```python
from build123d import *

# Parameters (mm, degrees)
F0_R     = 4.045
F0_R_2   = 1.575
F1_DEPTH = 5.44
F2_R     = 2.735
F3_DEPTH = 1.45
F4_R     = 2.375
F5_DEPTH = 2.5
F7_DEPTH = 2.4


with BuildPart() as f1:
    # F0 (on Front) → F1 (new body)
    with BuildSketch(Plane.XZ):
        Circle(F0_R)
        Circle(F0_R_2, mode=Mode.SUBTRACT)
    extrude(amount=F1_DEPTH)

    # F2 (on face) → F3 (cut)
    with BuildSketch(Plane.XZ.offset(5.44)):
        Circle(F2_R)
    extrude(amount=-F3_DEPTH, mode=Mode.SUBTRACT)

    # F4 (on face) → F5 (cut)
    with BuildSketch(Plane(origin=(0, 0, 0), x_dir=(-1, 0, 0), z_dir=(0, 1, 0))):
        Circle(F4_R)
    extrude(amount=-F5_DEPTH, mode=Mode.SUBTRACT)

    # F6 (on face) → F7 (join)
    with BuildSketch(Plane(origin=(0, 0, 0), x_dir=(-1, 0, 0), z_dir=(0, 1, 0))):
        with BuildLine():
            Line((1.4963533031, -0.268314818), (2.2665058776, -0.7096309653))
            ThreePointArc((2.2665058776, -0.7096309653), (2.3477197937, -0.3589383936), (2.375, 0))
            ThreePointArc((2.375, 0), (2.342926602, 0.3889986346), (2.247572684, 0.7674907361))
            Line((2.247572684, 0.7674907361), (1.4963533031, 0.266433459))
            ThreePointArc((1.4963533031, 0.266433459), (1.520064106, -0.0009406795), (1.4963533031, -0.268314818))
        make_face()
        with BuildLine():
            ThreePointArc((-0.7096309653, -2.2665058776), (0.0304393614, -2.3748049278), (0.7674907361, -2.247572684))
            Line((0.7674907361, -2.247572684), (0.266433459, -1.4963533031))
            ThreePointArc((0.266433459, -1.4963533031), (-0.0009406795, -1.520064106), (-0.268314818, -1.4963533031))
            Line((-0.268314818, -1.4963533031), (-0.7096309653, -2.2665058776))
        make_face()
        with BuildLine():
            ThreePointArc((-2.2665058776, 0.7096309653), (-2.3748049278, -0.0304393614), (-2.247572684, -0.7674907361))
            Line((-2.247572684, -0.7674907361), (-1.4963533031, -0.266433459))
            ThreePointArc((-1.4963533031, -0.266433459), (-1.520064106, 0.0009406795), (-1.4963533031, 0.268314818))
            Line((-1.4963533031, 0.268314818), (-2.2665058776, 0.7096309653))
        make_face()
        with BuildLine():
            ThreePointArc((0.7096309653, 2.2665058776), (-0.0304393614, 2.3748049278), (-0.7674907361, 2.247572684))
            Line((-0.7674907361, 2.247572684), (-0.266433459, 1.4963533031))
            ThreePointArc((-0.266433459, 1.4963533031), (0.0009406795, 1.520064106), (0.268314818, 1.4963533031))
            Line((0.268314818, 1.4963533031), (0.7096309653, 2.2665058776))
        make_face()
    extrude(amount=-F7_DEPTH)


solid = f1.part
```
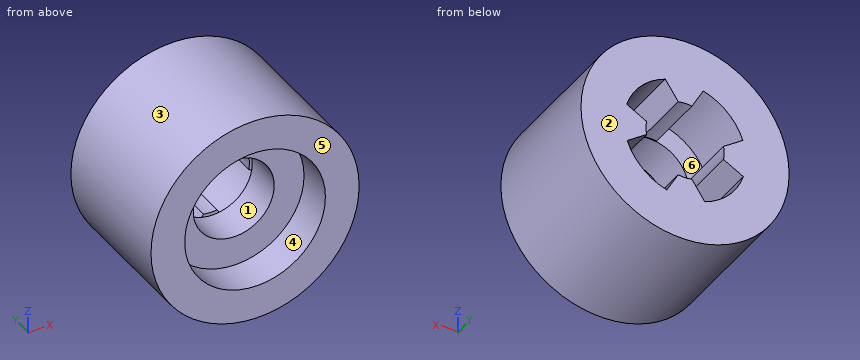
The listing builds one solid part. Answer for the finished solid, in the listing's coordinates (mm). Face numbers are marked on the shaded views. A direction names the side the tool comes from. Give positions to 0.01 mm unless a question says otherwise; leave off trailing zeros. Loops run counter-clockwise (first coordinate to the right, second up) from the corner with the lowest first, then second, coordinate; pieces in that order, holes last. Notation, with made-up numbers: M -2.5,82.5 L 15.5,82.5 A17 ccw 15.5,102.5 Z; hole C 28.5,-18 d8. An arc over 180 degrees is marked long. One line per item, written item: value.
Q1. Flat-ended cylindrical pins translate along their axes: P1, Ø3, axis at x = -2.5, y = -2.5, coming from the +Z side; P2, Ø1, axis at y = -4.5, z = -2, coming from the +X side; P3, Ø4.5, axis at x = 0, z = 0, coming from the -Y side. Find the tip coordinate at first contact, or state that the pin passes through.
Working result:
P1: stops at z = 3.92
P2: stops at x = 3.76
P3: stops at y = -3.99
Q2. A cutting plane is placed at B-B on x = 0. Determine the outline of the cut face in (y, z) (3 decimals).
Working result:
outline: M -5.44,-4.045 L 0,-4.045 L 0,-1.52 L -2.4,-1.52 L -2.4,-2.375 L -2.5,-2.375 L -2.5,-1.575 L -3.99,-1.575 L -3.99,-2.735 L -5.44,-2.735 Z; M -5.44,2.735 L -3.99,2.735 L -3.99,1.575 L -2.5,1.575 L -2.5,2.375 L -2.4,2.375 L -2.4,1.52 L 0,1.52 L 0,4.045 L -5.44,4.045 Z
Q3. For the marked faces 4, 5 and 6, determine the directions among +Z, -Z, +X, -X, +Y, -Y from which every point of the face is accessible in a straight line to the end or side of a thin tool.
Working result:
face 4: -Y
face 5: +Z, -Z, +X, -X, -Y
face 6: none
Q4. A cutting plane is placed at D-D on z = 2. Determine the outline of the cut face in (x, y), then the cut area to 3 significant figures.
Working result:
outline: M -3.52,-5.44 L -1.87,-5.44 L -1.87,-3.99 L 1.87,-3.99 L 1.87,-5.44 L 3.52,-5.44 L 3.52,0 L 1.28,0 L 1.28,-2.5 L -1.28,-2.5 L -1.28,0 L -3.52,0 Z; M -0.56,-2.4 L 0.6,-2.4 L 0.6,0 L -0.56,0 Z
area: 29.2 mm^2
Q5. Find the intervals of material crossed by line 1 (X direction, y = -0.8, z = -2); line 2 (Z direction, x = 0, y = -4.75) (3 decimals); line 3 (Z direction, x = 0, y = -1.55) (3 decimals), in increasing order. Write a range as from..to.
Working result:
line 1: x = -3.52..-1.28, -0.6..0.56, 1.28..3.52
line 2: z = -4.045..-2.735, 2.735..4.045
line 3: z = -4.045..-1.52, 1.52..4.045
Q6. A cutting plane is placed at A-A on z = 0. Determine the outline of the cut face in (x, y) (3 decimals), then the cut area to 3 significant figures.
Working result:
outline: M -4.045,-5.44 L -2.735,-5.44 L -2.735,-3.99 L -1.575,-3.99 L -1.575,-2.5 L -2.375,-2.5 L -2.375,-2.4 L -1.52,-2.4 L -1.52,0 L -4.045,0 Z; M 1.52,-2.4 L 2.375,-2.4 L 2.375,-2.5 L 1.575,-2.5 L 1.575,-3.99 L 2.735,-3.99 L 2.735,-5.44 L 4.045,-5.44 L 4.045,0 L 1.52,0 Z
area: 23.6 mm^2
Q7. Determine the mould class of the marked faces 1, 2 and 3 for opening direction X: +X half, -X half, draft (parallel to the pull), parting line (faces both ways), or undercut.
Working result:
face 1: undercut
face 2: draft
face 3: parting line
